The listing builds one solid part. Answer for the finished solid, in the listing's coordinates (mm). Give positions to 0.01 mm unless a question says otherwise; leave off trailing zeros. Return JSON: item names as keys, results as strings.
from build123d import *

# Parameters (mm, degrees)
F1_DEPTH = 1.5875


with BuildPart() as f1:
    # F0 (on Front) → F1 (new body)
    with BuildSketch(Plane.XZ):
        with BuildLine():
            Line((2.500466, 31.804252), (-3.337374, 31.804252))
            Line((-3.337374, 31.804252), (-17.745788, 20.465644))
            ThreePointArc((-17.745788, 20.465644), (-25.065561, 11.385533), (-27.594821, 0))
            ThreePointArc((-27.594821, 0), (-25.068458, -11.38136), (-17.745788, -20.453094))
            Line((-17.745788, -20.453094), (-29.64324, -32.335669))
            Line((-29.64324, -32.335669), (-23.884054, -32.335669))
            Line((-23.884054, -32.335669), (-14.268195, -24.034924))
            Line((-14.268195, -24.034924), (-22.640626, -32.335669))
            Line((-22.640626, -32.335669), (-17.583598, -32.335669))
            Line((-17.583598, -32.335669), (-7.984732, -24.03398))
            Line((-7.984732, -24.03398), (-16.352598, -32.335669))
            Line((-16.352598, -32.335669), (-11.296707, -32.335669))
            Line((-11.296707, -32.335669), (-1.655925, -23.997727))
            Line((-1.655925, -23.997727), (-10.060332, -32.335669))
            Line((-10.060332, -32.335669), (-4.89258, -32.335669))
            Line((-4.89258, -32.335669), (4.706284, -24.033981))
            Line((4.706284, -24.033981), (-3.66158, -32.335669))
            Line((-3.66158, -32.335669), (1.67275, -32.335669))
            Line((1.67275, -32.335669), (16.232245, -20.932899))
            ThreePointArc((16.232245, -20.932899), (23.431336, -11.561058), (25.880881, 0))
            ThreePointArc((25.880881, 0), (23.254287, 11.025444), (16.232245, 19.922092))
            Line((16.232245, 19.922092), (28.165267, 31.804252))
            Line((28.165267, 31.804252), (22.655676, 31.804252))
            Line((22.655676, 31.804252), (12.946506, 23.436493))
            Line((12.946506, 23.436493), (21.350084, 31.804252))
            Line((21.350084, 31.804252), (16.049387, 31.804252))
            Line((16.049387, 31.804252), (6.718841, 23.436493))
            Line((6.718841, 23.436493), (15.122419, 31.804252))
            Line((15.122419, 31.804252), (10.108952, 31.804252))
            Line((10.108952, 31.804252), (0.425895, 23.436493))
            Line((0.425895, 23.436493), (8.829473, 31.804252))
            Line((8.829473, 31.804252), (3.829063, 31.804252))
            Line((3.829063, 31.804252), (-5.903112, 23.436493))
            Line((-5.903112, 23.436493), (2.500466, 31.804252))
        make_face()
        with BuildLine():
            ThreePointArc((2.694642, 1.767532), (1.335932, 3.159091), (-0.427456, 3.979452))
            Line((-0.427456, 3.979452), (1.66349, 6.061486))
            ThreePointArc((1.66349, 6.061486), (4.845747, 3.680126), (6.347182, 0))
            ThreePointArc((6.347182, 0), (5.866074, -2.982653), (4.133003, -5.457355))
            Line((4.133003, -5.457355), (-23.493576, -30.398272))
            Line((-23.493576, -30.398272), (-25.043647, -30.398272))
            Line((-25.043647, -30.398272), (2.006969, -3.381483))
            ThreePointArc((2.006969, -3.381483), (2.71769, -2.601128), (3.157621, -1.64168))
            ThreePointArc((3.157621, -1.64168), (3.270361, 0.109673), (2.694642, 1.767532))
        make_face(mode=Mode.SUBTRACT)
        with BuildLine():
            ThreePointArc((7.720564, 0), (6.233101, 4.259643), (2.777397, 7.160541))
            Line((2.777397, 7.160541), (4.846783, 9.234832))
            ThreePointArc((4.846783, 9.234832), (8.986332, 5.381127), (10.72713, 0))
            ThreePointArc((10.72713, 0), (9.918057, -4.45281), (7.554526, -8.312322))
            Line((7.554526, -8.312322), (-17.312014, -30.398272))
            Line((-17.312014, -30.398272), (-18.735651, -30.398272))
            Line((-18.735651, -30.398272), (5.156565, -6.444786))
            ThreePointArc((5.156565, -6.444786), (7.161366, -3.509953), (7.720564, 0))
        make_face(mode=Mode.SUBTRACT)
        with BuildLine():
            ThreePointArc((8.497341, -9.450918), (11.293115, -5.096154), (12.192859, 0))
            ThreePointArc((12.192859, 0), (10.415009, 5.958783), (5.976826, 10.314284))
            Line((5.976826, 10.314284), (8.086616, 12.378573))
            ThreePointArc((8.086616, 12.378573), (13.188094, 7.082195), (15.167798, 0))
            ThreePointArc((15.167798, 0), (14.08092, -6.100532), (10.796622, -11.355165))
            Line((10.796622, -11.355165), (-11.222056, -30.398272))
            Line((-11.222056, -30.398272), (-12.51897, -30.398272))
            Line((-12.51897, -30.398272), (8.497341, -9.450918))
        make_face(mode=Mode.SUBTRACT)
        with BuildLine():
            Line((-5.040918, -30.398272), (-6.208889, -30.398272))
            Line((-6.208889, -30.398272), (12.476413, -11.58771))
            ThreePointArc((12.476413, -11.58771), (15.630392, -6.184107), (16.580828, 0))
            ThreePointArc((16.580828, 0), (14.510264, 7.649505), (9.189624, 13.522575))
            Line((9.189624, 13.522575), (11.269993, 15.594592))
            ThreePointArc((11.269993, 15.594592), (17.264531, 8.775118), (19.596276, 0))
            ThreePointArc((19.596276, 0), (17.840213, -8.751202), (12.435093, -15.854157))
            Line((12.435093, -15.854157), (-5.040918, -30.398272))
        make_face(mode=Mode.SUBTRACT)
        with BuildLine():
            ThreePointArc((20.982919, 0), (18.632523, 9.374038), (12.338778, 16.707912))
            Line((12.338778, 16.707912), (14.508339, 18.886948))
            ThreePointArc((14.508339, 18.886948), (21.382927, 10.519577), (23.954181, 0))
            ThreePointArc((23.954181, 0), (22.107779, -9.926357), (16.36753, -18.232456))
            Line((16.36753, -18.232456), (1.051465, -30.398272))
            Line((1.051465, -30.398272), (0, -30.398272))
            Line((0, -30.398272), (15.803264, -14.524432))
            ThreePointArc((15.803264, -14.524432), (19.78452, -7.758422), (20.982919, 0))
        make_face(mode=Mode.SUBTRACT)
        with BuildLine():
            Line((-16.761772, 18.597473), (-2.54207, 29.840623))
            Line((-2.54207, 29.840623), (-1.463471, 29.840623))
            Line((-1.463471, 29.840623), (-15.165877, 16.19467))
            ThreePointArc((-15.165877, 16.19467), (-20.625905, 8.914632), (-22.453522, 0))
            ThreePointArc((-22.453522, 0), (-20.242724, -9.692341), (-13.844848, -17.301303))
            Line((-13.844848, -17.301303), (-15.977073, -19.462374))
            ThreePointArc((-15.977073, -19.462374), (-23.020704, -10.845215), (-25.520603, 0))
            ThreePointArc((-25.520603, 0), (-23.326341, 10.327876), (-16.761772, 18.597473))
        make_face(mode=Mode.SUBTRACT)
        with BuildLine():
            Line((-13.788489, 15.40208), (3.616895, 29.840623))
            Line((3.616895, 29.840623), (4.808587, 29.840623))
            Line((4.808587, 29.840623), (-13.00357, 12.101851))
            ThreePointArc((-13.00357, 12.101851), (-16.74891, 6.552839), (-18.11982, 0))
            ThreePointArc((-18.11982, 0), (-16.169546, -7.988951), (-10.645506, -14.080904))
            Line((-10.645506, -14.080904), (-12.770631, -16.228664))
            ThreePointArc((-12.770631, -16.228664), (-18.934176, -9.136403), (-21.128622, 0))
            ThreePointArc((-21.128622, 0), (-19.154685, 8.509361), (-13.788489, 15.40208))
        make_face(mode=Mode.SUBTRACT)
        with BuildLine():
            Line((-9.702722, 13.103459), (9.771443, 29.809413))
            Line((9.771443, 29.809413), (11.151096, 29.809413))
            Line((11.151096, 29.809413), (-9.237427, 9.507794))
            ThreePointArc((-9.237427, 9.507794), (-12.491403, 5.236064), (-13.682904, 0))
            ThreePointArc((-13.682904, 0), (-12.084754, -6.314048), (-7.484162, -10.924453))
            Line((-7.484162, -10.924453), (-9.551929, -12.96554))
            ThreePointArc((-9.551929, -12.96554), (-14.800405, -7.409972), (-16.67208, 0))
            ThreePointArc((-16.67208, 0), (-14.772793, 7.394955), (-9.702722, 13.103459))
        make_face(mode=Mode.SUBTRACT)
        with BuildLine():
            Line((-8.06543, 8.717639), (15.884997, 29.83083))
            Line((15.884997, 29.83083), (17.292799, 29.83083))
            Line((17.292799, 29.83083), (-6.563151, 6.092896))
            ThreePointArc((-6.563151, 6.092896), (-8.545871, 3.328581), (-9.248127, 0))
            ThreePointArc((-9.248127, 0), (-7.954567, -4.625728), (-4.305757, -7.749323))
            Line((-4.305757, -7.749323), (-6.321113, -9.764679))
            ThreePointArc((-6.321113, -9.764679), (-10.718668, -5.748904), (-12.272709, 0))
            ThreePointArc((-12.272709, 0), (-11.158112, 4.836148), (-8.06543, 8.717639))
        make_face(mode=Mode.SUBTRACT)
        with BuildLine():
            Line((-5.838636, 4.71663), (22.008805, 29.83083))
            Line((22.008805, 29.83083), (23.542084, 29.83083))
            Line((23.542084, 29.83083), (-3.44265, 2.78213))
            ThreePointArc((-3.44265, 2.78213), (-4.742008, 0.626663), (-4.394693, -1.866074))
            ThreePointArc((-4.394693, -1.866074), (-3.019974, -3.523453), (-1.090547, -4.479523))
            Line((-1.090547, -4.479523), (-3.204506, -6.583116))
            ThreePointArc((-3.204506, -6.583116), (-6.527039, -3.994261), (-7.863931, 0))
            ThreePointArc((-7.863931, 0), (-7.341413, 2.568774), (-5.838636, 4.71663))
        make_face(mode=Mode.SUBTRACT)
    extrude(amount=F1_DEPTH)


solid = f1.part
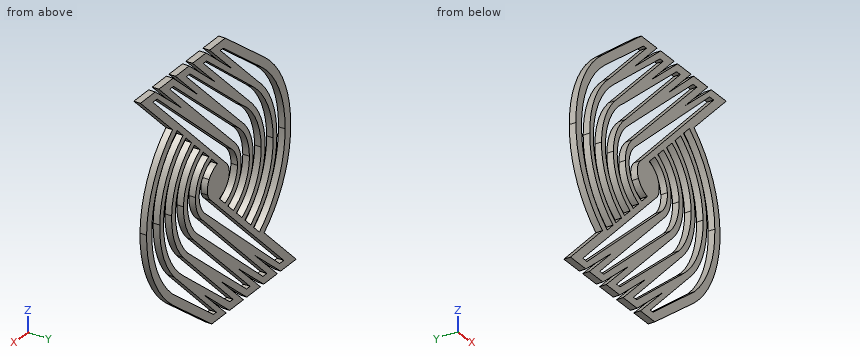
(1) Given pin 1 (0.7 mm diameter, centred on x = 16.5, y = -0.5, fed in from -Z); pin 2 (0.8 mm diameter, centred on x = -24, y = -1, fed in from +Z); pin 3 (0.8 mm diameter, centred on x = 22.5, y = -0.5, fed in from -Z), each flat-ended and moving along its own axis, determine where each tip first touches the part or whether it passes through.
Values follow:
{"pin 1": "z = -21", "pin 2": "z = 14.02", "pin 3": "z = -14.09"}
(2) Straight lines are drawn through the part: line 1 along X through (y, z) = (-1.3, 22); line 2 along X through (y, z) = (-0.7, -23.5); line 3 along Z through (x, y) = (21.5, -0.15). For each, find the intervals that lie inside material, in ascending order.
Values follow:
{"line 1": "-15.8 to -12.46, -9.34 to -5.83, -3.06 to 0.67, 3.31 to 7, 9.42 to 13.33, 15.73 to 18.32", "line 2": "-20.8 to -18.14, -15.85 to -11.86, -9.55 to -5.6, -3.25 to 0.64, 3.25 to 6.87, 9.74 to 12.95", "line 3": "-15.04 to -11.27, 10.28 to 14.1, 25.17 to 27.78, 29.37 to 30.81"}
(3) The part is cut by section A-A (y = -1.1). Give the number of separate pieces and of enclosed holes in the cut face, and give its area (3 significant figures).
Values follow:
{"separate pieces": "1", "enclosed holes": "10", "area": "1,340 mm²"}
